The figure shows three views and two pictorial views of one solid part (mm, origin at its lowest corner). Answer the questions. A direction names the side the tool comes from. Give positions to 0.01 mm unless a question says otherwise; leave off trailing zeros. Order: outer loops, then holes, each group sorted by start corner. A loop starts at its lowest first (then second) coordinate and runs counter-clockwise, first axis right, second up. Notation, with made-up numbers: (22, -20) - (31, -20) arc R34 cw to (31, 10) - close; hole circle Ø8 at (-25, 15). An arc over 180 degrees is marked (long way). Answer as CSV lines item,"result". Start each with the question number.
1. Section A-A on x = 18 is taken. Give the vertices of the cut face in (y, z), and give its area (3 significant figures).
2. Consider line 1 along Z through (x, y) = (35.1, 20); line 2 along X through (y, z) = (16, 6.25); line 3 along Y through (x, z) = (34, 2.25). Determine where each line is inside the solid, lowest interval first. Write a range as [from, to].
3. Section D-D on z = 1 is taken. Give the vertices of the cut face in (x, y), and give its area (3 significant figures).
4. Section B-B on y = 33 is taken. Give the vertices of the cut face in (x, z), and give its area (3 significant figures).
5. Section C-C on z = 8 is taken. Give the vertices of the cut face in (x, y).
6. Flat-ended cylindrical pins translate along their axes: pin 1 (1.7 mm diameter, centred on y = 7.5, z = 6.5, fed in from -X); pin 2 (10 mm diameter, centred on x = 25, y = 37.5, fed in from +Z); pin 3 (1.5 mm diameter, centred on y = 38, z = 2, fed in from -X); pin 4 (2.5 mm diameter, centred on y = 32.5, z = 1.5, fed in from +X). Find the tip coordinate at first contact, or state that the pin passes through.
7. Determine the mould class of the marked faces 1, 2 and 3 for opening direction X: +X half, -X half, draft (parallel to the pull), parting line (faces both ways), or undercut.
8. Which of the six approach directions +Z, -Z, +X, -X, +Y, -Y give full straight-line access (tool end or side, diameter ignored) to the marked faces 4, 5, 6 and 7?
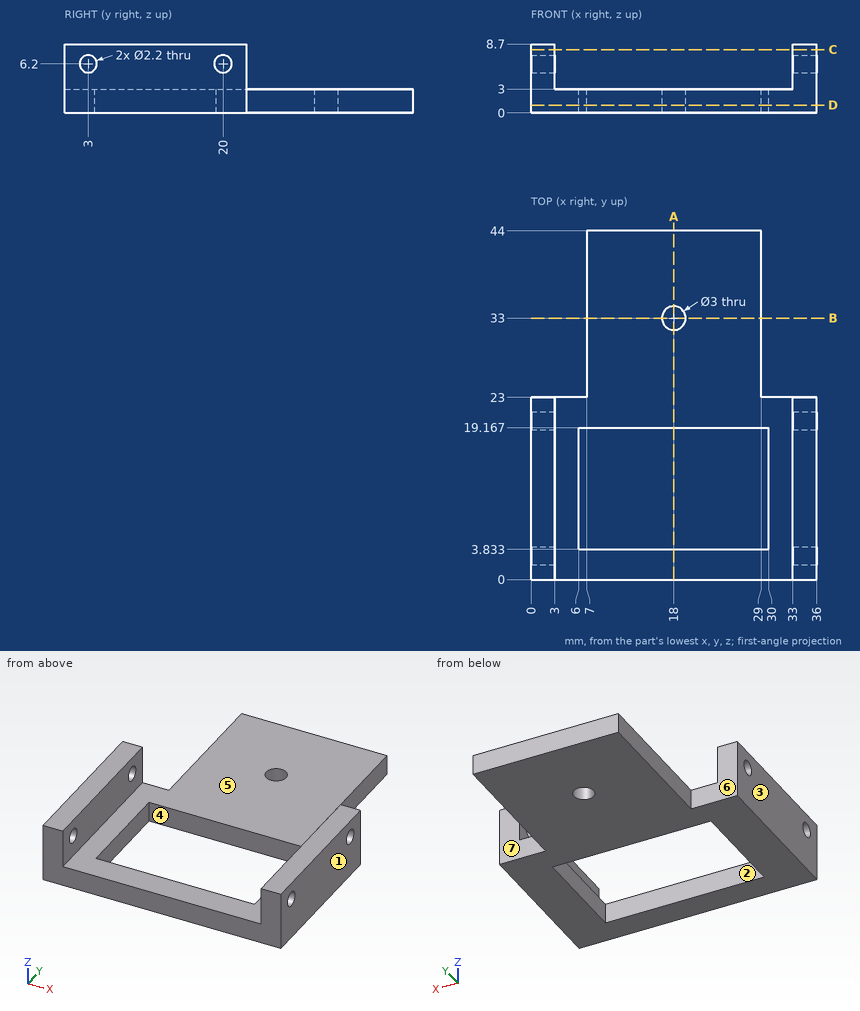
Checks:
1,outline,"(0, 0) - (3.83, 0) - (3.83, 3) - (0, 3) - close; (19.17, 0) - (31.5, 0) - (31.5, 3) - (19.17, 3) - close; (34.5, 0) - (44, 0) - (44, 3) - (34.5, 3) - close"
1,area,"77.0 mm²"
2,line 1,"z = [0, 5.1], [7.3, 8.7]"
2,line 2,"x = [0, 3], [33, 36]"
2,line 3,"y = [0, 23]"
3,outline,"(0, 0) - (36, 0) - (36, 23) - (29, 23) - (29, 44) - (7, 44) - (7, 23) - (0, 23) - close; hole (6, 3.83) - (30, 3.83) - (30, 19.17) - (6, 19.17) - close; hole circle Ø3 at (18, 33)"
3,area,"915 mm²"
4,outline,"(7, 0) - (16.5, 0) - (16.5, 3) - (7, 3) - close; (19.5, 0) - (29, 0) - (29, 3) - (19.5, 3) - close"
4,area,"57.0 mm²"
5,outline,"(0, 0) - (3, 0) - (3, 23) - (0, 23) - close; (33, 0) - (36, 0) - (36, 23) - (33, 23) - close"
6,pin 1,"stops at x = 0"
6,pin 2,"stops at z = 3"
6,pin 3,"stops at x = 7"
6,pin 4,"stops at x = 29"
7,face 1,"+X half"
7,face 2,"undercut"
7,face 3,"-X half"
8,face 4,"+Z, -Z"
8,face 5,"+Z, +Y, -Y"
8,face 6,"+Z, -Z, -X, +Y"
8,face 7,"+Z, -Z, +X, +Y"
